Could you check a few things on this drawing? It's one solid part, dimensions in mm from its lowest x, y, z. A direction names the side the tool comes from. Round coordinates to 2 decimals unless told otherwise and drop trailing zeros. Write each loop counter-clockwise with the first axis right and the second up, starting at its lowest first coordinate (ties: lowest second). Pieces come first, ordered by that corner, then holes. Notation, with made-up numbers: (-35, 23) - (1, 23) arc R3 ccw to (1, 27) - close; hole circle Ø8 at (5, 48). An arc over 180 degrees is marked (long way). Write item = value, one per line. Start each with the question number.
Item 1: If we section it at C-C (x = 1): Please give me the cut outline in (y, z).
Item 2: Which directions (+Z, -Z, +X, -X, +Y, -Y) give clear straight access to the entire face, cutting with the end or side of a thin tool? Please do the marked faces 1 and 2.
Item 3: If I drill on line 1 along Y through (x, z) = (5.05, 3); line 2 along Y through (x, z) = (3, 0.5); line 3 along Y through (x, z) = (5.5, 3.75), over which ranges is the centre line in solid material (lowest first)? Write a range as [from, to].
Item 4: Thinking about a two-plate mould opening in X: for the marked faces 3, 4 and 5, which applies, pulls with the +X half, pulls with the -X half, needs draft (parallel to the pull), parting line crosses it, or undercut?
Item 5: If we section it at A-A (z = 3): Please give me the cut outline in (x, y).
Item 6: For P1, Ø1.8, axis at y = 27, z = 3, coming from the +X side; P2, Ø0.8, axis at x = 3.5, z = 4, coming from the +Y side; P3, Ø1, axis at x = 4, y = 7, coming from the -Z side, each with a flat end and sliding along its axis, tell me the tip position at first contact or that it passes through.
Item 7: If we section it at D-D (z = 4.75): Please give me the cut outline in (x, y).
Item 8: If we section it at B-B (y = 27): Please give me the cut outline in (x, z).
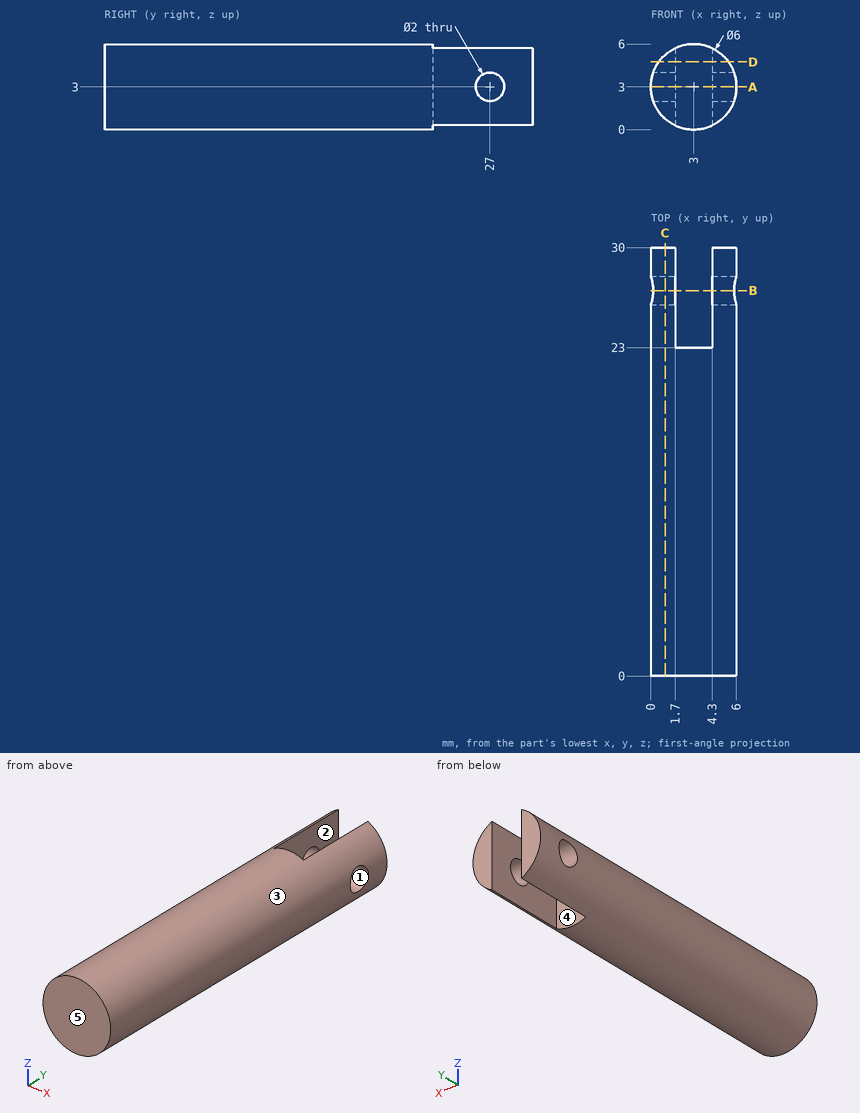
Reply:
q1.outline = (0, 0.76) - (30, 0.76) - (30, 5.24) - (0, 5.24) - close; hole circle Ø2 at (27, 3)
q2.face_1 = +X, -X
q2.face_2 = +Z, -Z, +Y
q3.line_1 = [0, 26], [28, 30]
q3.line_2 = [0, 23]
q3.line_3 = [0, 26.34], [27.66, 30]
q4.face_3 = parting line crosses it
q4.face_4 = undercut
q4.face_5 = needs draft
q5.outline = (0, 0) - (6, 0) - (6, 26) - (4.3, 26) - (4.3, 23) - (1.7, 23) - (1.7, 26) - (0, 26) - close; (0, 28) - (1.7, 28) - (1.7, 30) - (0, 30) - close; (4.3, 28) - (6, 28) - (6, 30) - (4.3, 30) - close
q6.P1 = through
q6.P2 = 23
q6.P3 = 0.04
q7.outline = (0.56, 0) - (5.44, 0) - (5.44, 30) - (4.3, 30) - (4.3, 23) - (1.7, 23) - (1.7, 30) - (0.56, 30) - close
q8.outline = (0.17, 2) arc R3 ccw to (1.7, 0.3) - (1.7, 2) - close; (0.17, 4) - (1.7, 4) - (1.7, 5.7) arc R3 ccw to start; (4.3, 0.3) arc R3 ccw to (5.83, 2) - (4.3, 2) - close; (4.3, 4) - (5.83, 4) arc R3 ccw to (4.3, 5.7) - close
